Read the model definition and answer for the solid it produces. Units are mm, in the model's axes. A direction names the side the tool comes from. Coordinates: 2 decimals unless noted, no trailing zeros. Write each loop counter-clockwise with the first axis right and the second up, starting at its lowest first coordinate (ties: lowest second). Pieces come first, ordered by that corner, then holes. Notation, with made-up numbers: (-12.75, 50.25) -> (42.25, 50.25) arc R15 cw to (42.25, 61.25) -> close; hole circle Ø4 at (41.25, -11.75). An arc over 180 degrees is marked (long way). Answer in a Markdown table with one row per item. Add a question column.
Item 1: Straight lines are drawn through the part: line 1 (X direction, y = -6, z = 55); line 2 (Z direction, x = -1, y = -6); line 3 (Y direction, x = 11, z = 66). For each, find the intervals that lie inside material, in ascending order. Write a range as from..to.
Item 2: Section B-B on y = -5.5 is taken. Write down the section's boundary in (x, z).
Item 3: Section C-C on z = 66.1 is taken. Write down the section's boundary in (x, y), then the cut area to 3 significant figures.
Item 4: Section D-D on x = 8.5 is taken. Write down the section's boundary in (y, z).
Item 5: Which of the six approach directions +Z, -Z, +X, -X, +Y, -Y give full straight-line access (tool end or side, diameter ignored) to faces 4 (the face through (-14, 1, 77.1)), 5 (the face through (-11.801, 1, 42)), 6 (the face through (-13, 8.169, 30)), 7 (the face through (-0.12, -5.352, 5.265)), 8 (the face through (-0.406, 4.635, 1.972))?
Item 6: For a pull along X with two mould halves and no side action, classify faces 1 (the face through (-2, 3, 4)), 2 (the face through (14.949, 1, 38)), 3 (the face through (-1, 1, 0)) as +X half, -X half, draft (parallel to the pull), parting line (faces both ways), or undercut.
Item 7: Section A-A on z = 31.5 is taken. Write down the section's boundary in (x, y), then the cut area to 3 significant figures.
Item 8: Given pin 1 Ø1.5 at (x, z) = (-1, 3.5) entering from -Y; pin 2 Ø4 at (y, z) = (0.67, 66.1) entering from +X; pin 3 Ø2 at (x, y) = (8, 1.5) entering from +Z, each flat-ended and moving along its own axis, determine where each tip first touches the part or whether it passes through.
```python
from build123d import *

# Parameters (mm, degrees)
SKETCH1_W           = 31.75
SKETCH1_H           = 15
BOSS_EXTRUDE1_DEPTH = 8
SKETCH2_W           = 5
SKETCH2_H           = 15
BOSS_EXTRUDE2_DEPTH = 69.1
SKETCH3_R           = 2.5
CUT_EXTRUDE1_DEPTH  = 69.1
SKETCH4_R           = 4
SKETCH4_R_2         = 2
CUT_EXTRUDE3_DEPTH  = 4
SKETCH5_R           = 1.5
CUT_EXTRUDE4_DEPTH  = 3


with BuildPart() as part:
    # Sketch1 → Boss-Extrude1 (new body)
    with BuildSketch(Plane.XY):
        with Locations((-0.926352113, 0.669031185)):
            Rectangle(SKETCH1_W, SKETCH1_H)
    extrude(amount=BOSS_EXTRUDE1_DEPTH)

    # Sketch2 → Boss-Extrude2 (add)
    with BuildSketch(Plane.XY.offset(8)):
        with Locations((-14.301352113, 0.669031185)):
            Rectangle(SKETCH2_W, SKETCH2_H)
        with Locations((12.448647887, 0.669031185)):
            Rectangle(SKETCH2_W, SKETCH2_H)
    extrude(amount=BOSS_EXTRUDE2_DEPTH)

    # Sketch3 → Cut-Extrude1 (cut)
    with BuildSketch(Plane(origin=(14.948647887, 0, 0), x_dir=(0, 0, -1), z_dir=(1, 0, 0))):
        with Locations(Location((-66.1, 0.669031185, 0), (0, 0, 90))):
            Circle(SKETCH3_R)
    extrude(amount=-CUT_EXTRUDE1_DEPTH, mode=Mode.SUBTRACT)

    # Sketch4 → Cut-Extrude3 (cut)
    with BuildSketch(Plane(origin=(0, 0, 0), x_dir=(-1, 0, 0), z_dir=(0, 0, -1))):
        with Locations((0.926352113, 0.669031185)):
            Circle(SKETCH4_R)
        with Locations((0.926352113, 0.669031185)):
            Circle(SKETCH4_R_2, mode=Mode.SUBTRACT)
    extrude(amount=-CUT_EXTRUDE3_DEPTH, mode=Mode.SUBTRACT)

    # Sketch5 → Cut-Extrude4 (cut)
    with BuildSketch(Plane.XZ.offset(6.830968815)):
        with Locations((-0.926352113, 4)):
            Circle(SKETCH5_R)
    extrude(amount=-CUT_EXTRUDE4_DEPTH, mode=Mode.SUBTRACT)


solid = part.part
```
Results below:
| question | item | result |
|---|---|---|
| 1 | line 1 | x = -16.8..-11.8, 9.95..14.95 |
| 1 | line 2 | z = 0..2.5, 5.5..8 |
| 1 | line 3 | y = -6.83..-1.83, 3.17..8.17 |
| 2 | outline | (-16.8, 0) -> (14.95, 0) -> (14.95, 77.1) -> (9.95, 77.1) -> (9.95, 8) -> (-11.8, 8) -> (-11.8, 77.1) -> (-16.8, 77.1) -> close; hole circle Ø3 at (-0.93, 4) |
| 3 | outline | (-16.8, -6.83) -> (-11.8, -6.83) -> (-11.8, -1.83) -> (-16.8, -1.83) -> close; (-16.8, 3.17) -> (-11.8, 3.17) -> (-11.8, 8.17) -> (-16.8, 8.17) -> close; (9.95, -6.83) -> (14.95, -6.83) -> (14.95, -1.83) -> (9.95, -1.83) -> close; (9.95, 3.17) -> (14.95, 3.17) -> (14.95, 8.17) -> (9.95, 8.17) -> close |
| 3 | area | 100 mm2 |
| 4 | outline | (-6.83, 0) -> (8.17, 0) -> (8.17, 8) -> (-6.83, 8) -> close |
| 5 | face 4 | +Z, +X, -X, +Y, -Y |
| 5 | face 5 | +Z, +Y, -Y |
| 5 | face 6 | +Z, -Z, +X, -X, +Y |
| 5 | face 7 | -Y |
| 5 | face 8 | -Z |
| 6 | face 1 | undercut |
| 6 | face 2 | +X half |
| 6 | face 3 | draft |
| 7 | outline | (-16.8, -6.83) -> (-11.8, -6.83) -> (-11.8, 8.17) -> (-16.8, 8.17) -> close; (9.95, -6.83) -> (14.95, -6.83) -> (14.95, 8.17) -> (9.95, 8.17) -> close |
| 7 | area | 150 mm2 |
| 8 | pin 1 | stops at y = -3.83 |
| 8 | pin 2 | passes through |
| 8 | pin 3 | stops at z = 8 |
